from build123d import *

# Parameters (mm, degrees)
SKETCH1_R           = 20.926913159
BOSS_EXTRUDE2_DEPTH = 30
SKETCH3_W           = 70
SKETCH3_H           = 41.853826318
BOSS_EXTRUDE3_DEPTH = 1.5
SKETCH4_R           = 3.25
CUT_EXTRUDE1_DEPTH  = 1.5


with BuildPart() as part:
    # Sketch1 → Boss-Extrude2 (new body)
    with BuildSketch(Plane(origin=(0, 0, 0), x_dir=(0, 0, -1), z_dir=(1, 0, 0))):
        Circle(SKETCH1_R)
    extrude(amount=BOSS_EXTRUDE2_DEPTH)

    # Sketch3 → Boss-Extrude3 (add)
    with BuildSketch(Plane.ZY):
        Rectangle(SKETCH3_W, SKETCH3_H)
    extrude(amount=-BOSS_EXTRUDE3_DEPTH)

    # Sketch4 → Cut-Extrude1 (cut)
    with BuildSketch(Plane.ZY):
        with Locations((28.25, 0)):
            Circle(SKETCH4_R)
        with Locations(Location((-28.25, 0, 0), (0, 0, 180))):
            Circle(SKETCH4_R)
    extrude(amount=-CUT_EXTRUDE1_DEPTH, mode=Mode.SUBTRACT)


solid = part.part
The model under review builds one solid part; all positions refer to its coordinate system, in mm. A direction names the side the tool comes from. Round coordinates to 2 decimals unless told otherwise and drop trailing zeros. Order: outer loops, then holes, each group sorted by start corner. A loop starts at its lowest first (then second) coordinate and runs counter-clockwise, first axis right, second up. Notation, with made-up numbers: (0, 88.25) -> (59, 88.25) arc R9 ccw to (59, 103.25) -> close; hole circle Ø2 at (46.25, 72). An arc over 180 degrees is marked (long way). Write item = value, one per line. Start each with the question number.
Item 1: Consider section A-A on y = 0. Write out the cut boundary in (x, z).
Item 2: Consider section D-D on z = 24. Write out the cut boundary in (x, y), plus the area to 3 significant figures.
Item 3: For faces 5 (the face through (1, 20.927, 0)), 6 (the face through (15.55, 6.29, -19.96)), list the 3-axis set-ups (+Z, -Z, +X, -X, +Y, -Y) from which the entire face can be reached by the end or side of a thin tool; tool diameter is ignored.
Item 4: For line 1 along Y through (x, z) = (0.7, 28.25); line 2 along X through (y, z) = (-4, -22.5); line 3 along Z through (x, y) = (14.5, 0.5), list the stretches that pass through material, from the lowest coordinate up.
Item 5: Clearance check with flat-ended pins moving along their axes: pin 1 Ø1.5 at (y, z) = (-12, 22.5) entering from -X; pin 2 Ø1.5 at (x, z) = (22.5, 20) entering from -Y; pin 3 Ø4 at (y, z) = (-4.5, 26) entering from +X; pin 4 Ø2 at (x, z) = (21.5, -5) entering from +Y. State where each tip first meets the part, or that it passes through.
Item 6: Consider section C-C on y = -14.5. Write out the cut boundary in (x, z), plus the area to 3 significant figures.
Item 7: Mouldability with a two-part tool opening along Y and no side actions: class faces 1 (the face through (1, -20.927, 0)), 2 (the face through (0.74, 0.98, 31.35)), 3 (the face through (1, 0, 35)), 4 (the face through (0.74, -0.98, -31.35)) as released by +Y, released by -Y, zero draft, split by the parting line, or undercut.
Item 8: Consider section B-B on z = -28.25. Write out the cut boundary in (x, y), plus the area to 3 significant figures.
Conclusion:
q1.outline = (0, -35) -> (1.5, -35) -> (1.5, -31.5) -> (0, -31.5) -> close; (0, -25) -> (1.5, -25) -> (1.5, -20.93) -> (30, -20.93) -> (30, 20.93) -> (1.5, 20.93) -> (1.5, 25) -> (0, 25) -> close; (0, 31.5) -> (1.5, 31.5) -> (1.5, 35) -> (0, 35) -> close
q2.outline = (0, -20.93) -> (1.5, -20.93) -> (1.5, 20.93) -> (0, 20.93) -> close
q2.area = 62.8 mm2
q3.face_5 = +Z, -Z, +X, -X, +Y
q3.face_6 = +X
q4.line_1 = -20.93 to -3.25, 3.25 to 20.93
q4.line_2 = 0 to 1.5
q4.line_3 = -20.92 to 20.92
q5.pin_1 = 0
q5.pin_2 = -8.21
q5.pin_3 = 1.5
q5.pin_4 = 20.54
q6.outline = (0, -35) -> (1.5, -35) -> (1.5, -15.09) -> (30, -15.09) -> (30, 15.09) -> (1.5, 15.09) -> (1.5, 35) -> (0, 35) -> close
q6.area = 965 mm2
q7.face_1 = released by -Y
q7.face_2 = undercut
q7.face_3 = zero draft
q7.face_4 = undercut
q8.outline = (0, -20.93) -> (1.5, -20.93) -> (1.5, -3.25) -> (0, -3.25) -> close; (0, 3.25) -> (1.5, 3.25) -> (1.5, 20.93) -> (0, 20.93) -> close
q8.area = 53.0 mm2
